Source: CAD feature listing. Evaluate the final solid. Frame: model axes, mm. A direction names the side the tool comes from. Coordinates: 2 decimals unless noted, no trailing zeros. Loops run counter-clockwise (first coordinate to the right, second up) from the corner with the lowest first, then second, coordinate; pieces in that order, holes last. Notation, with made-up numbers: (79.5, 11.5) - (87.5, 11.5) arc R21 cw to (87.5, 16.5) - close; hole circle Ø4 at (71, 36). An arc over 180 degrees is marked (long way). Use CSV: the item, a comma, the result in double quotes. Start each with the question number.
```python
from build123d import *

# Parameters (mm, degrees)
CUT_EXTRUDE1_DEPTH = 4


with BuildPart() as part:
    # Sketch2 → Revolve1 (revolve)
    with BuildSketch(Plane(origin=(0, 0, 0), x_dir=(0, 0, -1), z_dir=(1, 0, 0))):
        with BuildLine():
            Line((-12.5, 0), (-12.5, 4))
            Line((-12.5, 4), (-12.25, 4.25))
            Line((-12.25, 4.25), (-7.75, 4.25))
            Line((-7.75, 4.25), (-7.5, 4))
            Line((-7.5, 4), (-7.5, 2.75))
            ThreePointArc((-7.5, 2.75), (-7.426776695, 2.573223305), (-7.25, 2.5))
            Line((-7.25, 2.5), (11.980384758, 2.5))
            Line((11.980384758, 2.5), (12.5, 1.980384758))
            Line((12.5, 1.980384758), (12.5, 0))
            Line((12.5, 0), (-12.5, 0))
        make_face()
    revolve(axis=Axis((0, 0, -12.5), (0, 0, 1)))

    # Sketch3 → Cut-Extrude1 (cut)
    with BuildSketch(Plane.XY.offset(12.5)):
        Polygon((2, -1.154700538), (2, 1.154700538), (0, 2.309401077), (-2, 1.154700538), (-2, -1.154700538), (0, -2.309401077), align=None)
    extrude(amount=-CUT_EXTRUDE1_DEPTH, mode=Mode.SUBTRACT)

    # Cut-Extrude2 cone 1 section (through the dimple's axis) → Cut-Extrude2 (revolve, cut)
    with BuildSketch(Plane(origin=(0, 0, 12.5), x_dir=(0, -1, 0), z_dir=(1, 0, 0))):
        Polygon((0, 0), (2.482606158, 0), (0, 2.482606158), align=None)
    revolve(axis=Axis((0, 0, 12.5), (0, 0, -1)), mode=Mode.SUBTRACT)


solid = part.part
```
(1) Pin query (flat end, axial travel): pin 1 Ø2 at (y, z) = (-3, 0) entering from -X; pin 2 Ø1.2 at (x, y) = (-0.5, -1) entering from +Z; pin 3 Ø1.5 at (y, z) = (-2, -7.5) entering from +X. Return the tip coordinate at first contact, or that it passes through.
(2) Draft query along X for faces 1 (the cylindrical face through (2.44, -0.54, -2.5)), 2 (the flat face through (0.99, -1.74, 10.44)), 3 (the flat face through (-2, -2, 12.5)). Return one class per face: released by +X, released by -X, zero draft, split by the parting line, or undercut.
(3) Ray query, line 1 (X direction, y = 0, z = 9.75); line 2 (Y direction, x = -1, z = 9.25); line 3 (Z direction, x = 0.5, y = 0.75). Return the intervals inside material, ascending. Write a range as [from, to].
(4) Section A-A on y = 0. Output: boundary loops of the cut face in (x, z).
(5) Reachability of faces 4 (the flat face through (1.014, 1.724, 10.44)), 5 (the cylindrical face through (-3.584, 2.285, 9.968)), 6 (the flat face through (-1, 3, 7.5)) from +Z, -Z, +X, -X, +Y, -Y: full face, straight path, thin tool, end or side. Return the list, or none.
(6) Section B-B on z = -10. Output: boundary loops of the cut face in (x, y).
Solution:
1,pin 1,"stops at x = -1.5"
1,pin 2,"stops at z = 8.5"
1,pin 3,"stops at x = 2.17"
2,face 1,"split by the parting line"
2,face 2,"undercut"
2,face 3,"zero draft"
3,line 1,"x = [-4.25, -2], [2, 4.25]"
3,line 2,"y = [-4.13, -1.73], [1.73, 4.13]"
3,line 3,"z = [-12.5, 8.5]"
4,outline,"(-4.25, 7.75) - (-4, 7.5) - (-2.75, 7.5) arc R0.25 cw to (-2.5, 7.25) - (-2.5, -11.98) - (-1.98, -12.5) - (1.98, -12.5) - (2.5, -11.98) - (2.5, 7.25) arc R0.25 cw to (2.75, 7.5) - (4, 7.5) - (4.25, 7.75) - (4.25, 12.25) - (4, 12.5) - (2.48, 12.5) - (2, 12.02) - (2, 8.5) - (-2, 8.5) - (-2, 12.02) - (-2.48, 12.5) - (-4, 12.5) - (-4.25, 12.25) - close"
5,face 4,"+Z"
5,face 5,"+Z, -Z"
5,face 6,"-Z"
6,outline,"circle Ø5 at (0, 0)"
